Check sheet for the drawn part. Datum: minimum x, y, z corner. Units: mm. Give positions to 0.01 mm unless a question says otherwise; leave off trailing zeros. Write each loop counter-clockwise with the first axis right and the second up, starting at its lowest first coordinate (ties: lowest second). Pieces come first, ordered by that corner, then holes. Notation, with made-up numbers: (66.25, 3.25) -> (95.25, 3.25) arc R31 ccw to (95.25, 42.25) -> close; hole circle Ø7 at (89, -24). An arc over 180 degrees is marked (long way). Answer as CSV lines item,"result". Start each with the question number.
1) Sectioned sample at D-D on x = 1. Record the cut outline in (y, z), and give its area (3 significant figures).
2) Sectioned sample at C-C on y = 2.85. Record the cut outline in (x, z).
3) Mould release check, pull along Z, two halves, no side actions. Record for the marked faces 1, 2, 3 and 4: released by +Z, released by -Z, zero draft, split by the parting line, or undercut.
4) Material ranges on L1, parallel to Z at x = 1.75, y = 0.35 (1 decimal); L2, parallel to Z at x = 4.75, y = 1.8 (1 decimal); L3, parallel to X at y = 0.8, z = 2.5 (1 decimal), recorded low to high.
5) Sectioned sample at B-B on z = 3.75. Record the cut outline in (x, y).
6) Sectioned sample at A-A on x = 3.75. Record the cut outline in (y, z) (1 decimal).
7) Gauge pin test, flat end, axial feed: pin 1 Ø1 at (x, y) = (1.5, 1) entering from -Z (1 decimal). Record the tip position at first contact, or that the pin passes through.
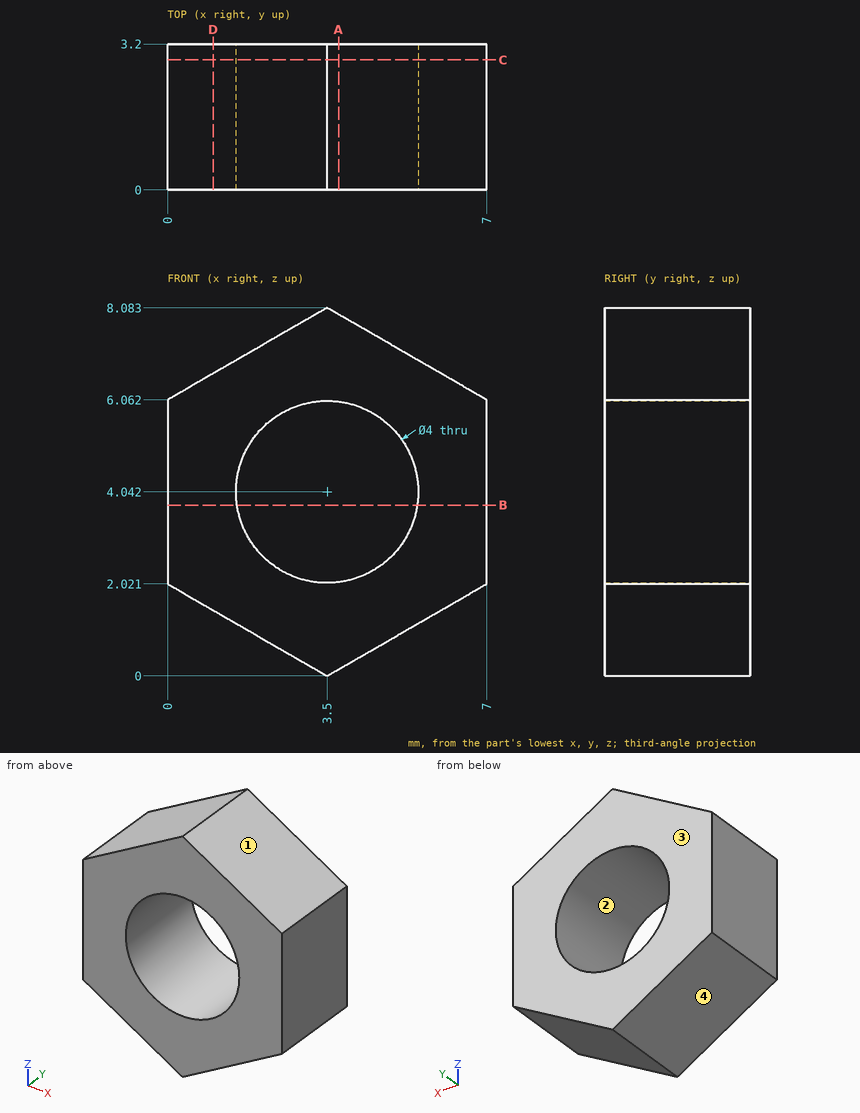
Ans:
1,outline,"(0, 1.44) -> (3.2, 1.44) -> (3.2, 6.64) -> (0, 6.64) -> close"
1,area,"16.6 mm²"
2,outline,"(0, 2.02) -> (3.5, 0) -> (7, 2.02) -> (7, 6.06) -> (3.5, 8.08) -> (0, 6.06) -> close; hole circle Ø4 at (3.5, 4.04)"
3,face 1,"released by +Z"
3,face 2,"undercut"
3,face 3,"zero draft"
3,face 4,"released by -Z"
4,L1,"z = 1 to 3.1, 5 to 7.1"
4,L2,"z = 0.7 to 2.5, 5.6 to 7.4"
4,L3,"x = 0 to 2.2, 4.8 to 7"
5,outline,"(0, 0) -> (1.52, 0) -> (1.52, 3.2) -> (0, 3.2) -> close; (5.48, 0) -> (7, 0) -> (7, 3.2) -> (5.48, 3.2) -> close"
6,outline,"(0, 0.1) -> (3.2, 0.1) -> (3.2, 2.1) -> (0, 2.1) -> close; (0, 6) -> (3.2, 6) -> (3.2, 7.9) -> (0, 7.9) -> close"
7,pin 1,"stops at z = 0.9"
